The model under review builds one solid part; all positions refer to its coordinate system, in mm. A direction names the side the tool comes from. Round coordinates to 2 decimals unless told otherwise and drop trailing zeros. Write each loop counter-clockwise with the first axis right and the second up, starting at its lowest first coordinate (ties: lowest second). Pieces come first, ordered by that corner, then holes. Notation, with made-up numbers: (14.25, 87) -> (41.25, 87) arc R9 ccw to (41.25, 104) -> close; hole circle Ø1 at (8.25, 62). An arc over 180 degrees is marked (long way). Answer in a Markdown table with one row per item. Add a question column.
Autodesk Inventor part; units mm, degrees
ref_plane "YZ Plane" through (0, 0, 0) normal (1, 0, 0) x (0, 1, 0)
ref_plane "XZ Plane" through (0, 0, 0) normal (0, 1, 0) x (-1, 0, 0)
ref_plane "XY Plane" through (0, 0, 0) normal (0, 0, 1) x (1, 0, 0)
sketch "Sketch1" plane through (0, 0, 0) normal (0, 1, 0) x (-1, 0, 0)
  line L0 (0, 0) -> (15, 0)
  line L1 (15, 0) -> (15, -10)
  line L2 (15, -10) -> (0, -10)
  line L3 (0, -10) -> (0, 0)
  line L4 (0, -5) -> (7.5006, -5)
  circle A0 centre (7.5006, -5) radius 0.4572
  line L5 (0, -5.254) -> (7.1205, -5.254)
  line L6 (0, -4.746) -> (7.1205, -4.746)
  dimension "d0" = 15
  dimension "d1" = 10
  dimension "d2" = 7.5006
  dimension "d3" = 0.9144
  dimension "d4" = 0.254
  dimension "d5" = 0.254
extrude "Extrusion1" add sketch "Sketch1" along normal blind 6.35 contours L0 L1 L2 L3 L5 A0 L6
sketch "Sketch2" plane through (-15, 0, 0) normal (0, 0, 1) x (1, 0, 0)
  line L0 (7.8795, 0) -> (15, 0)
  line L1 (15, 0) -> (8.65, 6.35)
  line L2 (15, 6.35) -> (7.8795, 6.35)
  line L3 (15, 0) -> (23.9803, 0) construction
  circle A0 centre (11.825, 3.175) radius 1.7526
  line L4 (15, 0) -> (0, 0)
  line L5 (0, 0) -> (6.35, 6.35)
  line L6 (7.0422, 6.35) -> (7.8795, 6.35)
  line L7 (0, 0) -> (8.9803, 0) construction
  circle A1 centre (3.175, 3.175) radius 1.7526
  dimension "d8" = 135
  dimension "d9" = 3.5052
  dimension "d10" = 45
  dimension "d11" = 3.5052
hole "Hole1" at (-11.825, 3.175, 0) direction (0, 0, -1) diameter 3.5052 end through all
hole "Hole2" at (-3.175, 3.175, 0) direction (0, 0, -1) diameter 3.5052 end through all
thread "Thread1"
thread "Thread2"
sketch "Sketch3" plane through (-15, 0, -10) normal (-1, 0, 0) x (0, 0, 1)
  line L0 (0, 6.35) -> (10, 6.35)
  line L1 (0, 6.35) -> (10, 0)
  circle A0 centre (5, 3.175) radius 0.508
  dimension "d30" = 1.016
extrude "Extrusion2" cut sketch "Sketch3" against normal blind 3.5001
properties part number "clamp(6-32)"
1. Add section C-C on z = -5. Write out the cut boundary in (x, y) (3 decimals).
2. Add section B-B on y = 4.5. Write out the cut boundary in (x, z).
3. Add section D-D on x = -7.5. Write out the cut boundary in (y, z), plus the area to 3 significant figures.
4. Tool access review of faces 5 (the cylindrical face through (-14.262, 2.866, -5.403)), 6 (the flat face through (-5.1, 3.1, -5.254)), 7 (the flat face through (0, 3, -8)): name each direction out of +Z, -Z, +X, -X, +Y, -Y from which nothing blocks a thin tool from reaching the whole face with its end or side.
5. Insertion check: pin 1 Ø2 at (x, y) = (-3.175, 3.175) entering from +Z; pin 2 Ø0.6 at (y, z) = (3.175, -5) entering from -X. Each pin has a flat end and moves straight along its axis. Give the tip position at first contact, or say it passes through.
6. For L1, parallel to Z at x = -5.25, y = 3.5; L2, parallel to X at y = 4.25, z = -2.75; L3, parallel to X at y = 3.5, z = -3.5, list the stretches that pass through material, from the lowest coordinate up.
7. Mouldability with a two-part tool opening along X and no side actions: class faces 1 (the flat face through (0, 3, -2)), 2 (the flat face through (-5.1, 3.1, -4.746)), 3 (the cylindrical face through (-7.958, 3.131, -4.984)), 4 (the cylindrical face through (-3.701, 1.503, -2.406)) as pulls with the +X half, pulls with the -X half, needs draft (parallel to the pull), parting line crosses it, or undercut.
8. Add section A-A on x = -5.5. Write out the cut boundary in (y, z), plus the area to 3 significant figures.
Filled in:
| question | item | result |
|---|---|---|
| 1 | outline | (-15, 0) -> (-7.958, 0) -> (-7.958, 6.35) -> (-15, 6.35) -> (-15, 3.683) -> (-13.502, 3.683) arc R1.753 cw (long way) to (-13.502, 2.667) -> (-15, 2.667) -> close |
| 2 | outline | (-15, -10) -> (-12.97, -10) -> (-12.97, 0) -> (-15, 0) -> close; (-10.68, -10) -> (-4.32, -10) -> (-4.32, -5.25) -> (-7.12, -5.25) arc R0.46 cw (long way) to (-7.12, -4.75) -> (-4.32, -4.75) -> (-4.32, 0) -> (-10.68, 0) -> close; (-2.03, -10) -> (0, -10) -> (0, -5.25) -> (-2.03, -5.25) -> close; (-2.03, -4.75) -> (0, -4.75) -> (0, 0) -> (-2.03, 0) -> close |
| 3 | outline | (0, -10) -> (6.35, -10) -> (6.35, -5.46) -> (0, -5.46) -> close; (0, -4.54) -> (6.35, -4.54) -> (6.35, 0) -> (0, 0) -> close |
| 3 | area | 57.7 mm² |
| 4 | face 5 | -X |
| 4 | face 6 | +X, +Y, -Y |
| 4 | face 7 | +Z, -Z, +X, +Y, -Y |
| 5 | pin 1 | through |
| 5 | pin 2 | x = -10.1 |
| 6 | L1 | -10 to -5.25, -4.75 to 0 |
| 6 | L2 | -15 to -13.21, -10.44 to -4.56, -1.79 to 0 |
| 6 | L3 | -15 to -13.55, -10.1 to -4.9, -1.45 to 0 |
| 7 | face 1 | pulls with the +X half |
| 7 | face 2 | needs draft |
| 7 | face 3 | undercut |
| 7 | face 4 | undercut |
| 8 | outline | (0, -10) -> (6.35, -10) -> (6.35, -5.25) -> (0, -5.25) -> close; (0, -4.75) -> (6.35, -4.75) -> (6.35, 0) -> (0, 0) -> close |
| 8 | area | 60.3 mm² |
